Input: part model. Units: mm. Frame: model coordinates. A direction names the side the tool comes from. Coordinates: 2 decimals unless noted, no trailing zeros. Loops run counter-clockwise (first coordinate to the right, second up) from the corner with the lowest first, then second, coordinate; pieces in that order, holes last.
Item 1: Pull-direction query (X, two-part tool) for faces 4 (the flat face through (49, 1, 34)), 5 (the flat face through (-45.776, 1.479, -21.7)), 6 (the cylindrical face through (-40.92, 1.48, -20.26)); classes: released by +X, released by -X, zero draft, split by the parting line, or undercut.
Item 2: Ray query, line 1 along X through (y, z) = (1.35, 15); line 2 along X through (y, z) = (1.3, 40.5); line 3 along Z through (x, y) = (22, 1.4). Return the intervals inside material, ascending.
Item 3: Section C-C on y = 2.05. Give the number of separate pieces and of enclosed holes in the cut face, and give its area (3 significant figures).
Item 4: Section B-B on x = 17.5. Return loops of the section in (y, z), and give its area (3 significant figures).
Item 5: Contact query for flat-ended pins moving along their axis: P1, Ø2, axis at x = 35.5, z = -17.5, coming from the -Y side; P2, Ø1.9, axis at x = -45, z = -49.5, coming from the -Y side; P3, Ø1.5, axis at x = -17, y = 1.5, coming from the +Z side; P4, Ø1, axis at y = 0.5, z = 31, coming from the -X side. Output: stop coordinate, or through.
Item 6: Section A-A on z = -35.5. Return loops of the section in (x, y), and give its area (3 significant figures).
Item 7: Reachability of faces 1 (the cylindrical face through (42.88, 1.48, 18.22)), 2 (the flat face through (-49, 1, -34)), 3 (the flat face through (-41, 1, 33)) from +Z, -Z, +X, -X, +Y, -Y: full face, straight path, thin tool, end or side. Return the list, or none.
```python
from build123d import *

# Parameters (mm, degrees)
SKETCH_1_R      = 1.6
SKETCH_1_R_2    = 2.25
SKETCH_1_R_3    = 1.05
SKETCH_1_W      = 73
SKETCH_1_H      = 36
EXTRUDE_2_DEPTH = 3


with BuildPart() as part:
    # 草图1 → 凸台-拉伸2 (new body)
    with BuildSketch(Plane(origin=(0, 0, 0), x_dir=(1, 0, 0), z_dir=(0, 1, 0))):
        with BuildLine():
            Line((41, 39.876524617), (41, 26.5))
            ThreePointArc((41, 26.5), (40.560660172, 25.439339828), (39.5, 25))
            ThreePointArc((39.5, 25), (38.085786438, 24.741657387), (36.854248689, 24))
            Line((36.854248689, 24), (-36.854248689, 24))
            ThreePointArc((-36.854248689, 24), (-38.085786438, 24.741657387), (-39.5, 25))
            ThreePointArc((-39.5, 25), (-40.560660172, 25.439339828), (-41, 26.5))
            Line((-41, 26.5), (-41, 39.876524617))
            ThreePointArc((-41, 39.876524617), (-45, 51.5), (-49, 39.876524617))
            Line((-49, 39.876524617), (-49, 27.037037037))
            ThreePointArc((-49, 27.037037037), (-48.630461799, 25.1505526), (-47.576470588, 23.54291939))
            Line((-47.576470588, 23.54291939), (-43.923529412, 19.803881957))
            ThreePointArc((-43.923529412, 19.803881957), (-42.869538201, 18.196248746), (-42.5, 16.30976431))
            Line((-42.5, 16.30976431), (-42.5, -16.30976431))
            ThreePointArc((-42.5, -16.30976431), (-42.869538201, -18.196248746), (-43.923529412, -19.803881957))
            Line((-43.923529412, -19.803881957), (-47.576470588, -23.54291939))
            ThreePointArc((-47.576470588, -23.54291939), (-48.630461799, -25.1505526), (-49, -27.037037037))
            Line((-49, -27.037037037), (-49, -39.876524617))
            ThreePointArc((-49, -39.876524617), (-45, -51.5), (-41, -39.876524617))
            Line((-41, -39.876524617), (-41, -26.5))
            ThreePointArc((-41, -26.5), (-40.560660172, -25.439339828), (-39.5, -25))
            ThreePointArc((-39.5, -25), (-38.085786438, -24.741657387), (-36.854248689, -24))
            Line((-36.854248689, -24), (36.854248689, -24))
            ThreePointArc((36.854248689, -24), (38.085786438, -24.741657387), (39.5, -25))
            ThreePointArc((39.5, -25), (40.560660172, -25.439339828), (41, -26.5))
            Line((41, -26.5), (41, -39.876524617))
            ThreePointArc((41, -39.876524617), (45, -51.5), (49, -39.876524617))
            Line((49, -39.876524617), (49, -27.037037037))
            ThreePointArc((49, -27.037037037), (48.630461799, -25.1505526), (47.576470588, -23.54291939))
            Line((47.576470588, -23.54291939), (43.923529412, -19.803881957))
            ThreePointArc((43.923529412, -19.803881957), (42.869538201, -18.196248746), (42.5, -16.30976431))
            Line((42.5, -16.30976431), (42.5, 16.30976431))
            ThreePointArc((42.5, 16.30976431), (42.869538201, 18.196248746), (43.923529412, 19.803881957))
            Line((43.923529412, 19.803881957), (47.576470588, 23.54291939))
            ThreePointArc((47.576470588, 23.54291939), (48.630461799, 25.1505526), (49, 27.037037037))
            Line((49, 27.037037037), (49, 39.876524617))
            ThreePointArc((49, 39.876524617), (45, 51.5), (41, 39.876524617))
        make_face()
        with Locations(Location((-39.5, 21, 0), (0, 0, 270))):
            Circle(SKETCH_1_R, mode=Mode.SUBTRACT)
        with Locations(Location((39.5, 21, 0), (0, 0, 270))):
            Circle(SKETCH_1_R, mode=Mode.SUBTRACT)
        with Locations(Location((39.5, -21, 0), (0, 0, 270))):
            Circle(SKETCH_1_R, mode=Mode.SUBTRACT)
        with Locations(Location((-39.5, -21, 0), (0, 0, 270))):
            Circle(SKETCH_1_R, mode=Mode.SUBTRACT)
        with Locations(Location((45, 45, 0), (0, 0, 270))):
            Circle(SKETCH_1_R_2, mode=Mode.SUBTRACT)
        with Locations(Location((45, 49.5, 0), (0, 0, 270))):
            Circle(SKETCH_1_R_3, mode=Mode.SUBTRACT)
        with Locations(Location((49.5, 45, 0), (0, 0, 270))):
            Circle(SKETCH_1_R_3, mode=Mode.SUBTRACT)
        with Locations(Location((45, 40.5, 0), (0, 0, 270))):
            Circle(SKETCH_1_R_3, mode=Mode.SUBTRACT)
        with Locations(Location((40.5, 45, 0), (0, 0, 270))):
            Circle(SKETCH_1_R_3, mode=Mode.SUBTRACT)
        with Locations(Location((40.5, -45, 0), (0, 0, 270))):
            Circle(SKETCH_1_R_3, mode=Mode.SUBTRACT)
        with Locations(Location((45, -40.5, 0), (0, 0, 270))):
            Circle(SKETCH_1_R_3, mode=Mode.SUBTRACT)
        with Locations(Location((49.5, -45, 0), (0, 0, 270))):
            Circle(SKETCH_1_R_3, mode=Mode.SUBTRACT)
        with Locations(Location((45, -49.5, 0), (0, 0, 270))):
            Circle(SKETCH_1_R_3, mode=Mode.SUBTRACT)
        with Locations(Location((45, -45, 0), (0, 0, 270))):
            Circle(SKETCH_1_R_2, mode=Mode.SUBTRACT)
        with Locations(Location((-45, -40.5, 0), (0, 0, 270))):
            Circle(SKETCH_1_R_3, mode=Mode.SUBTRACT)
        with Locations(Location((-40.5, -45, 0), (0, 0, 270))):
            Circle(SKETCH_1_R_3, mode=Mode.SUBTRACT)
        with Locations(Location((-45, -49.5, 0), (0, 0, 270))):
            Circle(SKETCH_1_R_3, mode=Mode.SUBTRACT)
        with Locations(Location((-49.5, -45, 0), (0, 0, 270))):
            Circle(SKETCH_1_R_3, mode=Mode.SUBTRACT)
        with Locations(Location((-45, -45, 0), (0, 0, 270))):
            Circle(SKETCH_1_R_2, mode=Mode.SUBTRACT)
        with Locations(Location((-40.5, 45, 0), (0, 0, 270))):
            Circle(SKETCH_1_R_3, mode=Mode.SUBTRACT)
        with Locations(Location((-45, 40.5, 0), (0, 0, 270))):
            Circle(SKETCH_1_R_3, mode=Mode.SUBTRACT)
        with Locations(Location((-49.5, 45, 0), (0, 0, 270))):
            Circle(SKETCH_1_R_3, mode=Mode.SUBTRACT)
        with Locations(Location((-45, 49.5, 0), (0, 0, 270))):
            Circle(SKETCH_1_R_3, mode=Mode.SUBTRACT)
        with Locations(Location((-45, 45, 0), (0, 0, 270))):
            Circle(SKETCH_1_R_2, mode=Mode.SUBTRACT)
        Rectangle(SKETCH_1_W, SKETCH_1_H, mode=Mode.SUBTRACT)
    extrude(amount=EXTRUDE_2_DEPTH)


solid = part.part
```
Results found:
1. face 4: released by +X
1. face 5: released by -X
1. face 6: undercut
2. line 1: x = -42.5 to -36.5, 36.5 to 42.5
2. line 2: x = -49.69 to -46.05, -43.95 to -40.31, 40.31 to 43.95, 46.05 to 49.69
2. line 3: z = -24 to -18, 18 to 24
3. separate pieces: 1
3. enclosed holes: 25
3. area: 2,390 mm2
4. outline: (0, -24) - (3, -24) - (3, -18) - (0, -18) - close; (0, 18) - (3, 18) - (3, 24) - (0, 24) - close
4. area: 36.0 mm2
5. P1: stops at y = 0
5. P2: passes through
5. P3: stops at z = 24
5. P4: stops at x = -49
6. outline: (-49, 0) - (-41, 0) - (-41, 3) - (-49, 3) - close; (41, 0) - (49, 0) - (49, 3) - (41, 3) - close
6. area: 48.0 mm2
7. face 1: +X, +Y, -Y
7. face 2: -X, +Y, -Y
7. face 3: +Y, -Y
